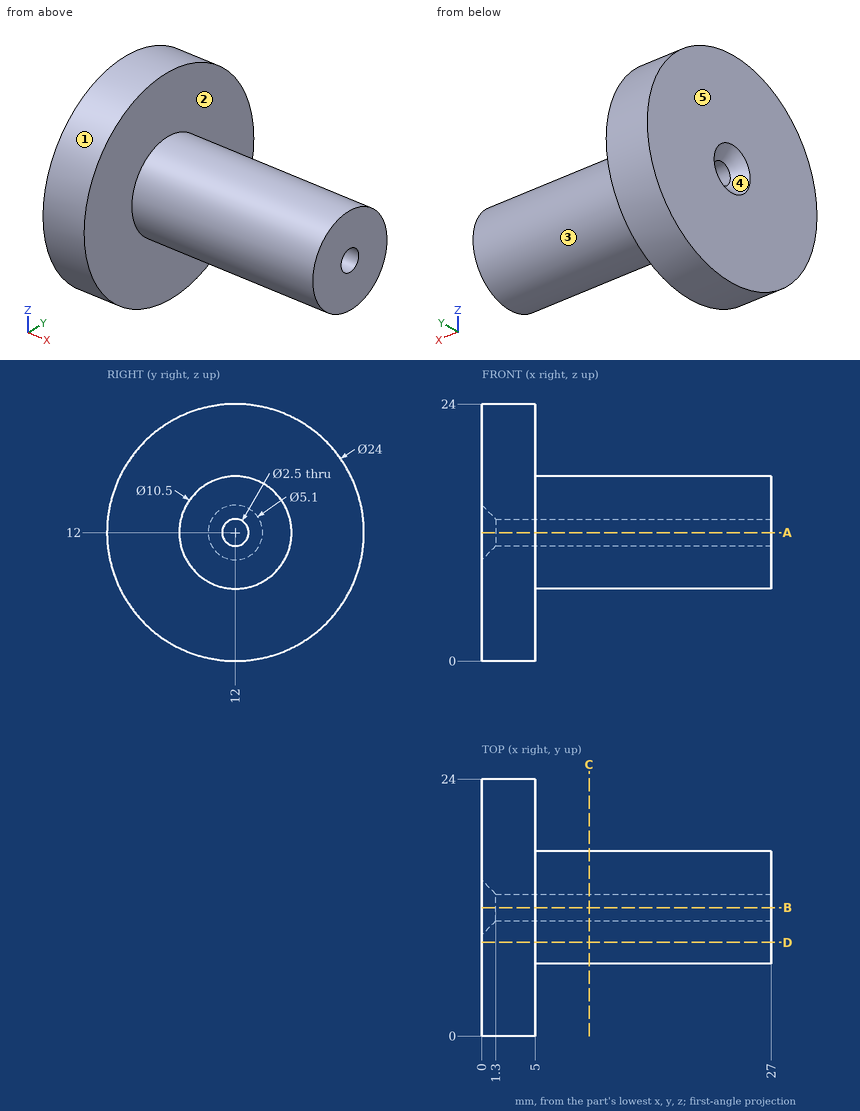
Design review of the part shown in the three views and the two pictorial views. Dimensions are in mm from the part's minimum x, y and z. A direction names the side the tool comes from. Give positions to 0.01 mm unless a question says otherwise; leave off trailing zeros. Write each loop counter-clockwise with the first axis right and the second up, starting at its lowest first coordinate (ties: lowest second). Pieces come first, ordered by that corner, then holes. Notation, with made-up numbers: M 71.25,70.25 L 109.25,70.25 A22 cw 109.25,99.25 Z; hole C 32.25,-31 d8. An arc over 180 degrees is marked long. One line per item, written item: value.
1) For line 1 (Y direction, x = 7.5, z = 12); line 2 (X direction, y = 4, z = 4.5), list the stretches that pass through material, from the lowest coordinate up. Write a range as from..to.
Results are:
line 1: y = 6.75..10.75, 13.25..17.25
line 2: x = 0..5
2) For the marked faces 1 and 2, list the 3-axis set-ups (+Z, -Z, +X, -X, +Y, -Y) from which the entire face can be reached by the end or side of a thin tool; tool diameter is ignored.
Results are:
face 1: +X, -X
face 2: +X
3) The part is to be moulded in two halves that separate along Z. For the marked faces 3, 4 and 5, say which applies: +Z half, -Z half, draft (parallel to the pull), parting line (faces both ways), or undercut.
Results are:
face 3: parting line
face 4: undercut
face 5: draft
4) Take a section at D-D, the plane y = 8.75. Write out the cut boundary in (x, z), then the cut area to 3 significant figures.
Results are:
outline: M 0,0.45 L 5,0.45 L 5,7.88 L 27,7.88 L 27,16.12 L 5,16.12 L 5,23.55 L 0,23.55 Z
area: 297 mm²
5) Take a section at A-A, the plane z = 12. Write out the cut boundary in (x, y).
Results are:
outline: M 0,0 L 5,0 L 5,6.75 L 27,6.75 L 27,10.75 L 1.3,10.75 L 0,9.45 Z; M 0,14.55 L 1.3,13.25 L 27,13.25 L 27,17.25 L 5,17.25 L 5,24 L 0,24 Z
6) Take a section at C-C, the plane x = 10. Write out the cut boundary in (y, z).
Results are:
outline: C 12,12 d10.5; hole C 12,12 d2.5
7) For P1, Ø1, axis at y = 11, z = 4, coming from the +X side; P2, Ø10, axis at x = 6, y = 17.5, coming from the -Z side; P3, Ø1.5, axis at x = 10.5, z = 12, coming from the +Y side, all flat-tipped, find the tip position at first contact; note any pin that passes through.
Results are:
P1: stops at x = 5
P2: stops at z = 0.02
P3: stops at y = 17.25
